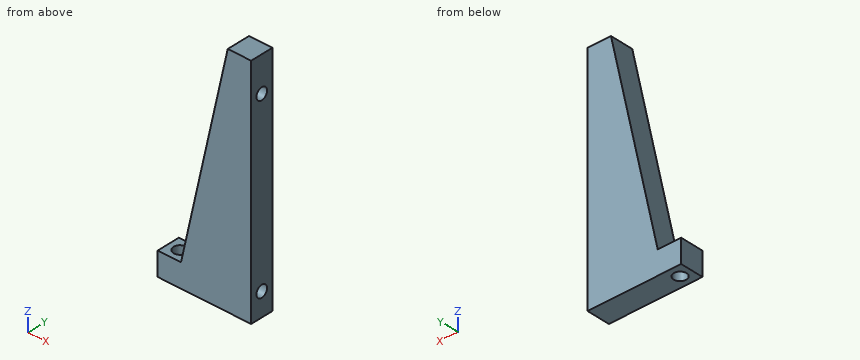
from build123d import *

# Parameters (mm, degrees)
F1_DEPTH = 10
F2_R     = 2.75
F3_DEPTH = 25
F4_R     = 2.5
F5_DEPTH = 10


with BuildPart() as f1:
    # F0 (on Front) → F1 (new body)
    with BuildSketch(Plane.XZ):
        Polygon((0, 10), (0, 0), (40, 0), (40, 100), (30, 100), (10, 10), align=None)
    extrude(amount=F1_DEPTH)

    # F2 (on face) → F3 (cut)
    with BuildSketch(Plane.XY.offset(10)):
        with Locations((5, -5)):
            Circle(F2_R)
    extrude(amount=-F3_DEPTH, mode=Mode.SUBTRACT)

    # F4 (on face) → F5 (cut)
    with BuildSketch(Plane.YZ.offset(40)):
        with Locations((-5, 85)):
            Circle(F4_R)
        with Locations((-5, 10)):
            Circle(F4_R)
    extrude(amount=-F5_DEPTH, mode=Mode.SUBTRACT)


solid = f1.part
Read the model definition and answer for the solid it produces. Units are mm, in the model's axes. Coordinates: 2 decimals unless noted, no trailing zeros. Order: outer loops, then holes, each group sorted by start corner. A loop starts at its lowest first (then second) coordinate and runs counter-clockwise, first axis right, second up. Notation, with made-up numbers: (-23, -3.5) -> (-19, -3.5) arc R27 ccw to (-19, 17.5) -> close; hole circle Ø6 at (5.25, -24.75). An arc over 180 degrees is marked (long way). Answer as a JSON object with one key per item and string values.
1) A cutting plane is placed at A-A, the plane x = 5. Determine the outline of the cut face in (y, z), plus the area to 3 significant figures.
Model answer:
{"outline": "(-10, 0) -> (-7.75, 0) -> (-7.75, 10) -> (-10, 10) -> close; (-2.25, 0) -> (0, 0) -> (0, 10) -> (-2.25, 10) -> close", "area": "45.0 mm²"}
2) A cutting plane is placed at C-C, the plane x = 32.5. Determine the outline of the cut face in (y, z), plus the area to 3 significant figures.
Model answer:
{"outline": "(-10, 0) -> (0, 0) -> (0, 100) -> (-10, 100) -> close; hole circle Ø5 at (-5, 10); hole circle Ø5 at (-5, 85)", "area": "961 mm²"}
3) A cutting plane is placed at B-B, the plane y = -3.5. Determine the outline of the cut face in (x, z).
Model answer:
{"outline": "(0, 0) -> (2.7, 0) -> (2.7, 10) -> (0, 10) -> close; (7.3, 0) -> (40, 0) -> (40, 8) -> (30, 8) -> (30, 12) -> (40, 12) -> (40, 83) -> (30, 83) -> (30, 87) -> (40, 87) -> (40, 100) -> (30, 100) -> (10, 10) -> (7.3, 10) -> close"}
4) Consider line 1 along Z through (x, y) = (37.75, -5); line 2 along Y through (x, z) = (5, 3); line 3 along Y through (x, z) = (6.5, 5). Determine where each line is inside the solid, lowest interval first. Write a range as from..to.
Model answer:
{"line 1": "z = 0..7.5, 12.5..82.5, 87.5..100", "line 2": "y = -10..-7.75, -2.25..0", "line 3": "y = -10..-7.3, -2.7..0"}
5) A cutting plane is placed at D-D, the plane z = 85. Determine the outline of the cut face in (x, y), plus the area to 3 significant figures.
Model answer:
{"outline": "(26.67, -10) -> (40, -10) -> (40, -7.5) -> (30, -7.5) -> (30, -2.5) -> (40, -2.5) -> (40, 0) -> (26.67, 0) -> close", "area": "83.3 mm²"}
6) Each of these flat-tipped pins is pushed along its axis until it touches: pin 1 (3 mm diameter, centred on y = -5, z = 85, fed in from -X); pin 2 (1 mm diameter, centred on y = -6, z = 28.5, fed in from -X); pin 3 (3 mm diameter, centred on x = 5, y = -6.5, fed in from +Z). Where does it stop, or does it pass through?
Model answer:
{"pin 1": "stops at x = 26.33", "pin 2": "stops at x = 14", "pin 3": "stops at z = 10"}
